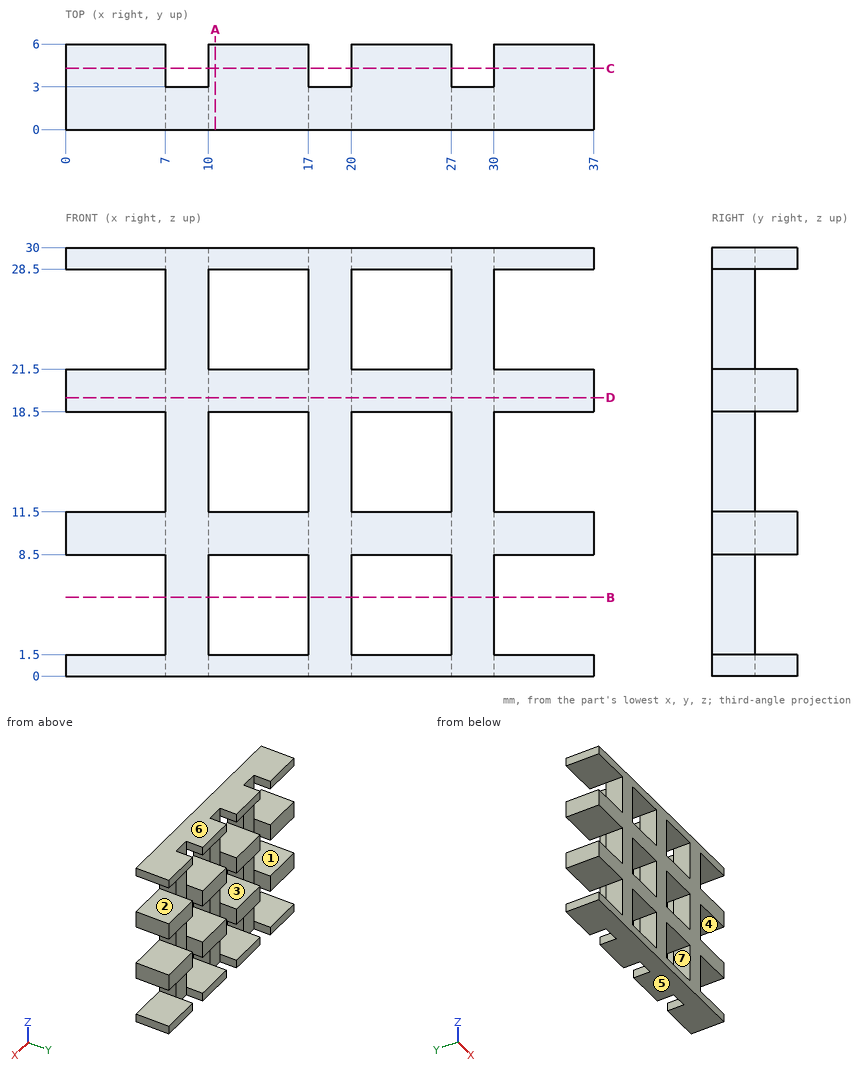
Job drawing, mm, ordinate dimensions from the low corner. One solid piece. A direction names the side the tool comes from. Coordinates: 2 decimals unless noted, no trailing zeros. Write each loop counter-clockwise with the first axis right and the second up, starting at its lowest first coordinate (ties: lowest second). Pieces come first, ordered by that corner, then holes. Notation, with made-up numbers: M 2,21.25 L 29,21.25 A17 cw 29,44.25 Z; hole C -27.5,4.5 d5. An arc over 180 degrees is marked long. Answer as a JSON object with one key per item and string values. Group by question number.
1) Wall check: line 1 (X direction, y = 2.55, z = 13.5); line 2 (Z direction, x = 10.5, y = 0.5); line 3 (Y direction, x = 18, z = 26.5). Give the ranges that are in metal, low to high. Write a range as from..to.
2) Saw through at C-C (y = 4.3). Give the number of separate pieces and of enclosed holes in the cut face, plus the area to 3 significant figures.
3) Pin check, flat tips, straight feed: pin 1 Ø2.5 at (y, z) = (5, 9.5) entering from -X; pin 2 Ø0.9 at (y, z) = (1.5, 15) entering from +X; pin 3 Ø3.5 at (y, z) = (2, 14) entering from -X. Stop position of each tip, or through.
4) Saw through at A-A (x = 10.5). Write the cut outline in (y, z).
5) Saw through at B-B (z = 5.5). Write the cut outline in (x, y).
6) Saw through at D-D (z = 19.5). Write the cut outline in (x, y), plus the area to 3 significant figures.
7) Mould opens along Z. For the marked faces 4, 5, 6 and 7 say: +Z half, -Z half, draft (parallel to the pull), parting line (faces both ways), or undercut.
8) Tool access for the marked faces 1, 2 and 3: list every direction of +Z, -Z, +X, -X, +Y, -Y with a clear straight run to the whole face (end or side of a thin tool).
Values follow:
{
 "1": {"line 1": "x = 7..10, 17..20, 27..30", "line 2": "z = 0..1.5, 8.5..11.5, 18.5..21.5, 28.5..30", "line 3": "y = 0..3"},
 "2": {"separate pieces": "16", "enclosed holes": "0", "area": "252 mm2"},
 "3": {"pin 1": "stops at x = 0", "pin 2": "stops at x = 30", "pin 3": "stops at x = 7"},
 "4": {"outline": "M 0,0 L 6,0 L 6,1.5 L 0,1.5 Z; M 0,8.5 L 6,8.5 L 6,11.5 L 0,11.5 Z; M 0,18.5 L 6,18.5 L 6,21.5 L 0,21.5 Z; M 0,28.5 L 6,28.5 L 6,30 L 0,30 Z"},
 "5": {"outline": "M 7,0 L 10,0 L 10,3 L 7,3 Z; M 17,0 L 20,0 L 20,3 L 17,3 Z; M 27,0 L 30,0 L 30,3 L 27,3 Z"},
 "6": {"outline": "M 0,0 L 37,0 L 37,6 L 30,6 L 30,3 L 27,3 L 27,6 L 20,6 L 20,3 L 17,3 L 17,6 L 10,6 L 10,3 L 7,3 L 7,6 L 0,6 Z", "area": "195 mm2"},
 "7": {"face 4": "undercut", "face 5": "-Z half", "face 6": "+Z half", "face 7": "undercut"},
 "8": {"face 1": "-X, +Y, -Y", "face 2": "+X, +Y, -Y", "face 3": "+Y, -Y"}
}
